from build123d import *

# Parameters (mm, degrees)
F0_W     = 96.76984
F0_H     = 49.842296
F1_DEPTH = 25.4
F2_W     = 96.76984
F2_H     = 44.49164
F3_DEPTH = 21.844
F5_DEPTH = 64.516
F6_R     = 9.073272
F7_DEPTH = 25.4


with BuildPart() as f1:
    # F0 (on Top) → F1 (new body)
    with BuildSketch(Plane.XY):
        with Locations((-4.372131, -2.331802)):
            Rectangle(F0_W, F0_H)
    extrude(amount=F1_DEPTH)

    # F2 (on face) → F3 (join)
    with BuildSketch(Plane.XZ.offset(27.25295)):
        with Locations((-4.372131, 3.15418)):
            Rectangle(F2_W, F2_H)
        Polygon((17.488524, -39.786395), (44.012789, -19.09164), (-52.757051, -19.09164), (-25.649834, -39.786395), align=None)
    extrude(amount=-F3_DEPTH)

    # F4 (on face) → F5 (cut)
    with BuildSketch(Plane(origin=(0, 22.589346, 0), x_dir=(-1, 0, 0), z_dir=(0, 1, 0))):
        Polygon((25.066886, 14.719509), (15.739672, 25.4), (-13.990819, 25.4), (-22.735082, 14.719509), align=None)
    extrude(amount=-F5_DEPTH, mode=Mode.SUBTRACT)

    # F6 (on face) → F7 (cut)
    with BuildSketch(Plane(origin=(0, 0, 0), x_dir=(1, 0, 0), z_dir=(0, 0, -1))):
        with Locations((0, -9.686902)):
            Circle(F6_R)
    extrude(amount=-F7_DEPTH, mode=Mode.SUBTRACT)


solid = f1.part
Geometry check sheet. Reference: the model listing, model coordinates, mm. A direction names the side the tool comes from. Give positions to 0.01 mm unless a question says otherwise; leave off trailing zeros. Loops run counter-clockwise (first coordinate to the right, second up) from the corner with the lowest first, then second, coordinate; pieces in that order, holes last. Notation, with made-up numbers: (-29, 32) -> (-15, 32) arc R12 ccw to (-15, 52) -> close; hole circle Ø8 at (-31.75, 33). An arc over 180 degrees is marked (long way). Answer in a Markdown table with one row per item. Add a question column.
1) Gauge pin test, flat ends, axial feed: P1, Ø8.5, axis at x = 19, y = 9.5, coming from the -Z side; P2, Ø4, axis at x = -6.5, y = 2.5, coming from the +Z side; P3, Ø8, axis at y = 14.5, z = -4.5, coming from the -X side; P4, Ø20, axis at x = -20, z = -28, coming from the +Y side. Record the tip position at first contact, or that the pin passes through.
2) Draft check along X on faces 1 (the face through (-39.393, -16.484, -29.294)), 2 (the face through (-4, -16, -39.786)), 3 (the face through (18.302, -1.983, 20.135)). Enter one of: pulls with the +X half, pulls with the -X half, needs draft (parallel to the pull), parting line crosses it, or undercut.
3) Set-up check for faces 4 (the face through (-5, -5.409, -20)), 5 (the face through (-35, -2, 25.4)), 6 (the face through (-1, -2, 14.72)): record each of +Z, -Z, +X, -X, +Y, -Y from which the full face is reachable in a straight line by a thin tool's end or side.
4) Cross-section at D-D on y = 17. Record the boundary of the cut face in (x, z).
5) Cross-section at C-C on z = -17. Record the boundary of the cut face in (x, y), and give its area (3 significant figures).
6) Cross-section at A-A on x = 0. Record the boundary of the cut face in (y, z), and give its area (3 significant figures).
7) Cross-section at B-B on y = -22.5. Record the boundary of the cut face in (x, z).
8) Material ranges on probe 1 along Y at (x, z) = (0, 9); probe 2 along Y at (x, z) = (2, -24); probe 3 along X at (y, z) = (8.5, 3), recorded low to high. Write a range as from..to.
Outcome:
| question | item | result |
|---|---|---|
| 1 | P1 | stops at z = 0 |
| 1 | P2 | stops at z = 14.72 |
| 1 | P3 | passes through |
| 1 | P4 | stops at y = -5.41 |
| 2 | face 1 | pulls with the -X half |
| 2 | face 2 | needs draft |
| 2 | face 3 | undercut |
| 3 | face 4 | -Z, +X, -X, +Y |
| 3 | face 5 | +Z, +X, -X, +Y, -Y |
| 3 | face 6 | +Y, -Y |
| 4 | outline | (-52.76, 0) -> (-5.37, 0) -> (-5.37, 14.72) -> (-25.07, 14.72) -> (-15.74, 25.4) -> (-52.76, 25.4) -> close; (5.37, 0) -> (44.01, 0) -> (44.01, 25.4) -> (13.99, 25.4) -> (22.74, 14.72) -> (5.37, 14.72) -> close |
| 5 | outline | (-52.76, -27.25) -> (44.01, -27.25) -> (44.01, -5.41) -> (-52.76, -5.41) -> close |
| 5 | area | 2,110 mm^2 |
| 6 | outline | (-27.25, -39.79) -> (-5.41, -39.79) -> (-5.41, 0) -> (0.61, 0) -> (0.61, 14.72) -> (-27.25, 14.72) -> close; (18.76, 0) -> (22.59, 0) -> (22.59, 14.72) -> (18.76, 14.72) -> close |
| 6 | area | 1,340 mm^2 |
| 7 | outline | (-52.76, -19.09) -> (-25.65, -39.79) -> (17.49, -39.79) -> (44.01, -19.09) -> (44.01, 25.4) -> (13.99, 25.4) -> (22.74, 14.72) -> (-25.07, 14.72) -> (-15.74, 25.4) -> (-52.76, 25.4) -> close |
| 8 | probe 1 | y = -27.25..0.61, 18.76..22.59 |
| 8 | probe 2 | y = -27.25..-5.41 |
| 8 | probe 3 | x = -52.76..-9, 9..44.01 |
